Study the drawing (mm; zero at the part's minimum x, y, z) and answer. Give positions to 0.01 mm unless a question says otherwise; leave off trailing zeros. Write each loop counter-clockwise with the first axis right and the second up, starting at its lowest first coordinate (ties: lowest second). Pieces come first, ordered by that corner, then holes.
1) Find section A-A (z = 11). Determine the outline of the cut face in (x, y).
2) Given pin 1 Ø2 at (x, z) = (5, 11) entering from -Y, flat-ended and moving along its own axis, determine where the tip first touches the part or whether it passes through.
3) Find section C-C (x = 5). Determine the outline of the cut face in (y, z).
4) Determine the mould class of the marked faces 1, 2 and 3 for opening direction Z: pulls with the +Z half, pulls with the -Z half, needs draft (parallel to the pull), parting line crosses it, or undercut.
5) Straight lines are drawn through the part: probe 1 along X at (y, z) = (1.55, 11); probe 2 along Z at (x, y) = (35, 2.45); probe 3 along Z at (x, y) = (6, 0.7). For each, find the intervals that lie inside material, in ascending order.
6) Find section B-B (y = 1.6). Determine the outline of the cut face in (x, z), plus the area to 3 significant figures.
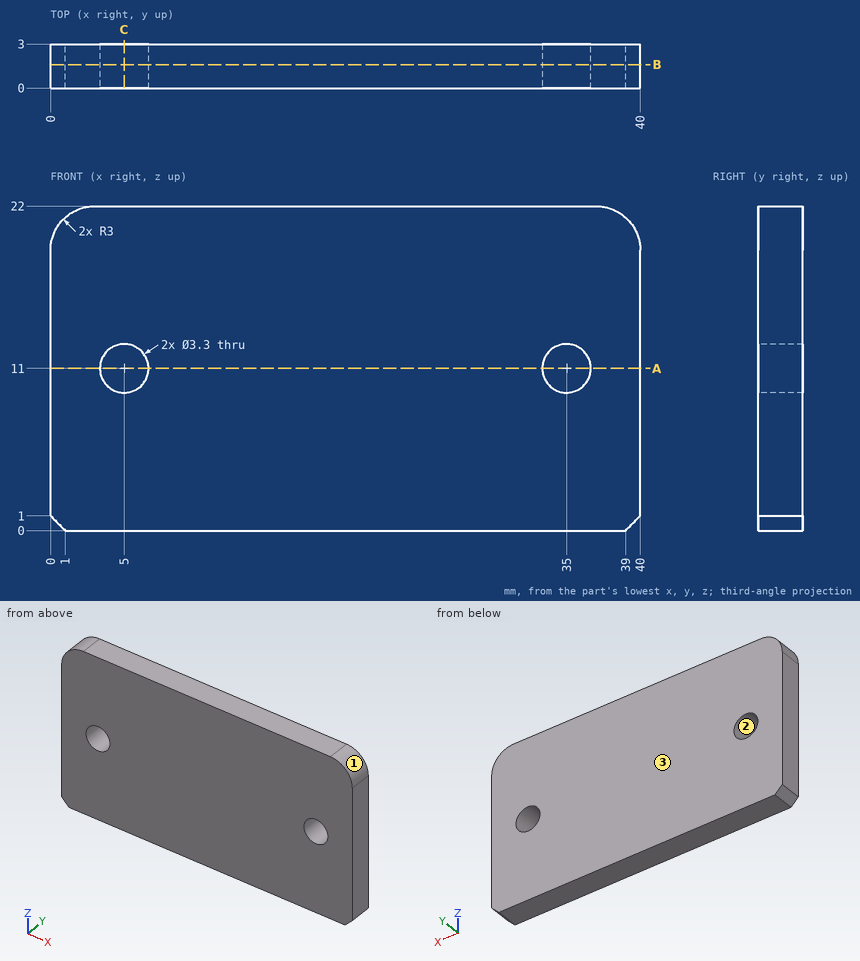
Results:
1. outline: (0, 0) - (3.35, 0) - (3.35, 3) - (0, 3) - close; (6.65, 0) - (33.35, 0) - (33.35, 3) - (6.65, 3) - close; (36.65, 0) - (40, 0) - (40, 3) - (36.65, 3) - close
2. pin 1: passes through
3. outline: (0, 0) - (3, 0) - (3, 9.35) - (0, 9.35) - close; (0, 12.65) - (3, 12.65) - (3, 22) - (0, 22) - close
4. face 1: pulls with the +Z half
4. face 2: undercut
4. face 3: needs draft
5. probe 1: x = 0 to 3.35, 6.65 to 33.35, 36.65 to 40
5. probe 2: z = 0 to 9.35, 12.65 to 22
5. probe 3: z = 0 to 9.69, 12.31 to 22
6. outline: (0, 1) - (1, 0) - (39, 0) - (40, 1) - (40, 19) arc R3 ccw to (37, 22) - (3, 22) arc R3 ccw to (0, 19) - close; hole circle Ø3.3 at (5, 11); hole circle Ø3.3 at (35, 11)
6. area: 858 mm2
